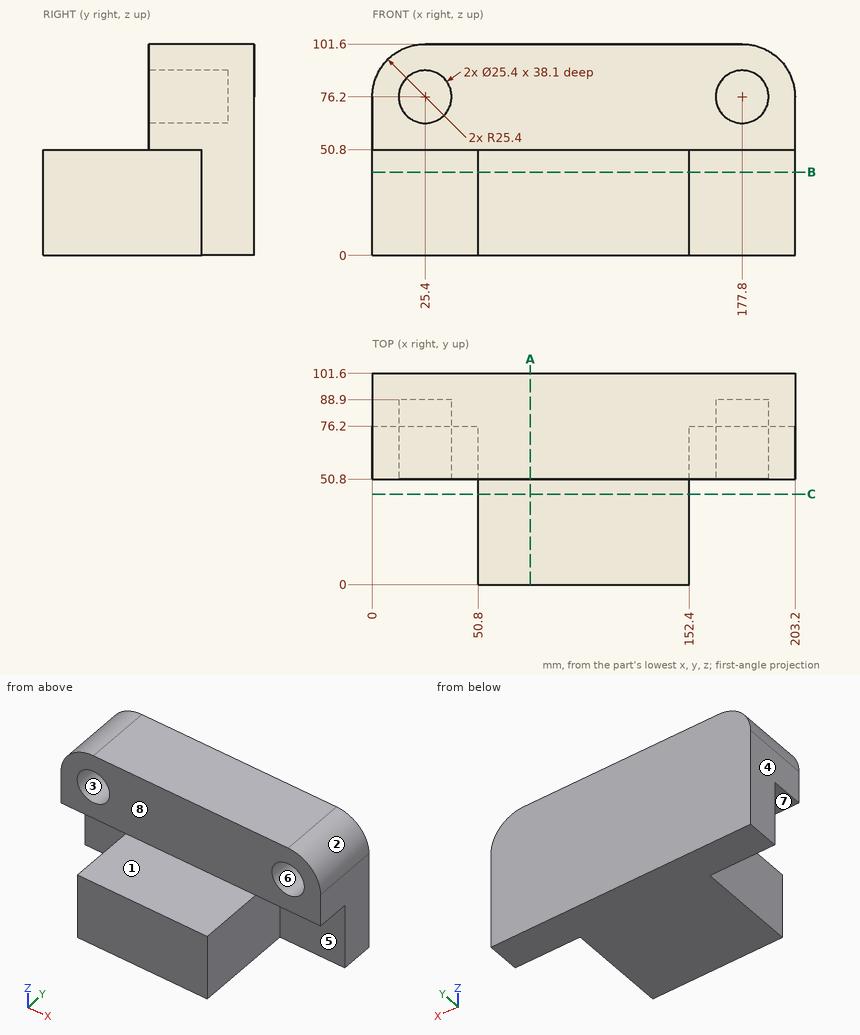
Job drawing, mm, ordinate dimensions from the low corner. One solid piece. A direction names the side the tool comes from. Round coordinates to 2 decimals unless told otherwise and drop trailing zeros. Loops run counter-clockwise (first coordinate to the right, second up) from the corner with the lowest first, then second, coordinate; pieces in that order, holes last. Notation, with made-up numbers: (53, 78.5) -> (91, 78.5) arc R18 cw to (91, 106.5) -> close; hole circle Ø5 at (77, 69.25). An arc over 180 degrees is marked (long way). Use CSV: the item, a comma, the result in double quotes. Start each with the question number.
Q1. Which spindle directions (+Z, -Z, +X, -X, +Y, -Y) get a long thin tool onto all of the face, cutting with end or side? Do the marked faces 4, 5, 6, 7 and 8. Say none if no direction does.
Q2. Flat gauge pins, fed straight in: pin 1 Ø3 at (y, z) = (19, 45.5) entering from +X; pin 2 Ø12 at (y, z) = (39.5, 32) entering from -X; pin 3 Ø15 at (x, z) = (29.5, 16.5) entering from -Y. Where does each tip first touch, or does it go through?
Q3. Saw through at B-B on z = 40. Give the cut face in (x, y), and give its area (3 significant figures).
Q4. Mould opens along X. For the marked faces 1, 2 and 3 say: +X half, -X half, draft (parallel to the pull), parting line (faces both ways), or undercut.
Q5. Saw through at A-A on x = 76. Give the cut face in (y, z), and give its area (3 significant figures).
Q6. Saw through at C-C on y = 43.5. Give the cut face in (x, z).
Q7. Drill centre lines: L1, parallel to Z at x = 177.8, y = 73.5; L2, parallel to Z at x = 56, y = 32; L3, parallel to Y at x = 166, z = 90. Where is each one in solid material? Low to high.
Solutions:
1,face 4,"+Z, -Z, -X, +Y, -Y"
1,face 5,"-Z, +X, -Y"
1,face 6,"-Y"
1,face 7,"-Z, -X, -Y"
1,face 8,"+Z, +X, -X, -Y"
2,pin 1,"stops at x = 152.4"
2,pin 2,"stops at x = 50.8"
2,pin 3,"stops at y = 76.2"
3,outline,"(0, 76.2) -> (50.8, 76.2) -> (50.8, 0) -> (152.4, 0) -> (152.4, 76.2) -> (203.2, 76.2) -> (203.2, 101.6) -> (0, 101.6) -> close"
3,area,"12,900 mm^2"
4,face 1,"draft"
4,face 2,"+X half"
4,face 3,"undercut"
5,outline,"(0, 0) -> (101.6, 0) -> (101.6, 101.6) -> (50.8, 101.6) -> (50.8, 50.8) -> (0, 50.8) -> close"
5,area,"7,740 mm^2"
6,outline,"(50.8, 0) -> (152.4, 0) -> (152.4, 50.8) -> (50.8, 50.8) -> close"
7,L1,"z = 50.8 to 63.5, 88.9 to 101.6"
7,L2,"z = 0 to 50.8"
7,L3,"y = 50.8 to 101.6"
